from build123d import *

# Parameters (mm, degrees)
SKETCH1_R           = 14
BOSS_EXTRUDE1_DEPTH = 4
SKETCH2_R           = 13
SKETCH2_R_2         = 12
BOSS_EXTRUDE2_DEPTH = 6
SKETCH2_3_R         = 12
SKETCH2_3_R_2       = 10
BOSS_EXTRUDE3_DEPTH = 7
SKETCH2_4_R         = 10
BOSS_EXTRUDE4_DEPTH = 3
SKETCH3_R           = 9.5
BOSS_EXTRUDE5_DEPTH = 4
FILLET1_R           = 8
SKETCH5_R           = 1.5
CUT_EXTRUDE1_DEPTH  = 3.5
SKETCH6_R           = 5.1
CUT_EXTRUDE2_DEPTH  = 4.2


with BuildPart() as part:
    # Sketch1 → Boss-Extrude1 (new body)
    with BuildSketch(Plane(origin=(0, 0, 0), x_dir=(1, 0, 0), z_dir=(0, 1, 0))):
        with Locations(Location((0, 0, 0), (0, 0, 270))):
            Circle(SKETCH1_R)
    extrude(amount=BOSS_EXTRUDE1_DEPTH)

    # Sketch2 → Boss-Extrude2 (add)
    with BuildSketch(Plane(origin=(0, 4, 0), x_dir=(1, 0, 0), z_dir=(0, 1, 0))):
        with Locations(Location((0, 0, 0), (0, 0, 270))):
            Circle(SKETCH2_R)
        with Locations(Location((0, 0, 0), (0, 0, 270))):
            Circle(SKETCH2_R_2, mode=Mode.SUBTRACT)
    extrude(amount=BOSS_EXTRUDE2_DEPTH)

    # Sketch2<3> → Boss-Extrude3 (add)
    with BuildSketch(Plane(origin=(0, 4, 0), x_dir=(1, 0, 0), z_dir=(0, 1, 0))):
        with Locations(Location((0, 0, 0), (0, 0, 90))):
            Circle(SKETCH2_3_R)
        with Locations(Location((0, 0, 0), (0, 0, 90))):
            Circle(SKETCH2_3_R_2, mode=Mode.SUBTRACT)
    extrude(amount=BOSS_EXTRUDE3_DEPTH)

    # Sketch2<4> → Boss-Extrude4 (add)
    with BuildSketch(Plane(origin=(0, 4, 0), x_dir=(1, 0, 0), z_dir=(0, 1, 0))):
        with Locations(Location((0, 0, 0), (0, 0, 90))):
            Circle(SKETCH2_4_R)
    extrude(amount=BOSS_EXTRUDE4_DEPTH)

    # Sketch3 → Boss-Extrude5 (add)
    with BuildSketch(Plane(origin=(0, 7, 0), x_dir=(1, 0, 0), z_dir=(0, 1, 0))):
        with Locations(Location((0, 0, 0), (0, 0, 270))):
            Circle(SKETCH3_R)
    extrude(amount=BOSS_EXTRUDE5_DEPTH)

    # Fillet1
    # the kernel refuses this fillet: 8 mm, written as the material it takes off along each edge
    with BuildSketch(Plane(origin=(0, 11, 0), x_dir=(0, 0, 1), z_dir=(-1, 0, 0))) as fillet1_piece_1:
        with BuildLine():
            CenterArc((2.57179677, -8), FILLET1_R, 30, 60)
            Line((2.57179677, 0), (2.57179677, 0.16))
            Line((2.57179677, 0.16), (9.5, 0.16))
            Line((9.5, 0.16), (9.66, 0))
            ThreePointArc((9.66, 0), (9.66, -2), (9.638564065, -3.92))
            Line((9.638564065, -3.92), (9.5, -4))
        make_face()
    revolve(axis=Axis((0, 11, 0), (0, 1, 0)), mode=Mode.SUBTRACT)

    # Sketch5 → Cut-Extrude1 (cut)
    with BuildSketch(Plane(origin=(0, 11, 0), x_dir=(1, 0, 0), z_dir=(0, 1, 0))):
        with Locations(Location((0, 6.5, 0), (0, 0, 270))):
            Circle(SKETCH5_R)
        with Locations(Location((6.5, 0, 0), (0, 0, 270))):
            Circle(SKETCH5_R)
        with Locations(Location((0, -6.5, 0), (0, 0, 270))):
            Circle(SKETCH5_R)
        with Locations(Location((-6.5, 0, 0), (0, 0, 270))):
            Circle(SKETCH5_R)
    extrude(amount=-CUT_EXTRUDE1_DEPTH, mode=Mode.SUBTRACT)

    # Sketch6 → Cut-Extrude2 (cut)
    with BuildSketch(Plane.XZ):
        with Locations(Location((0, 0, 0), (0, 0, 270))):
            Circle(SKETCH6_R)
    extrude(amount=-CUT_EXTRUDE2_DEPTH, mode=Mode.SUBTRACT)


solid = part.part
Read the model definition and answer for the solid it produces. Units are mm, in the model's axes. A direction names the side the tool comes from. Round coordinates to 2 decimals unless told otherwise and drop trailing zeros. Use a Markdown table: item, result.
(1) Which of the six approach directions +Z, -Z, +X, -X, +Y, -Y give full straight-line access (tool end or side, diameter ignored) to faces 1 (the cylindrical face through (-7.91, 6.958, -10.316)), 2 (the flat face through (0, 11, 0)), 3 (the flat face through (0, 4.2, 0))?
Reported:
| item | result |
|---|---|
| face 1 | +Y |
| face 2 | +Z, -Z, +X, -X, +Y |
| face 3 | -Y |
(2) Each of these flat-tipped pins is pushed along its axis until it touches: pin 1 Ø2.5 at (x, z) = (0.5, 6) entering from +Y; pin 2 Ø5 at (x, z) = (6.5, 0) entering from +Y; pin 3 Ø9 at (x, z) = (0, 0) entering from -Y. Where does it stop, or does it pass through?
Reported:
| item | result |
|---|---|
| pin 1 | y = 10.69 |
| pin 2 | y = 10.87 |
| pin 3 | y = 4.2 |
(3) The mould has two halves that part along Z. Classify faces 4 (the cylindrical face through (-13.67, 1.97, -3.03)), 5 (the flat face through (-9, 11, 5)), 6 (the flat face through (0, 7.5, -7)): released by +Z, released by -Z, zero draft, split by the parting line, or undercut.
Reported:
| item | result |
|---|---|
| face 4 | split by the parting line |
| face 5 | zero draft |
| face 6 | undercut |
(4) Straight lines are drawn through the part: line 1 along X through (y, z) = (9.95, 0); line 2 along X through (y, z) = (8.4, 0); line 3 along Y through (x, z) = (-4, -8.75). For each, find the intervals that lie inside material, in ascending order. Write a range as [from, to].
Reported:
| item | result |
|---|---|
| line 1 | [-13, -10], [-5, 5], [10, 13] |
| line 2 | [-13, -10], [-8.47, -8], [-5, 5], [8, 8.47], [10, 13] |
| line 3 | [0, 7] |
